```python
from build123d import *

# Parameters (mm, degrees)
SKETCH_1_R               = 2
EXTRUDE_1_DEPTH          = 4
SKETCH_1_3_W             = 3
SKETCH_1_3_H             = 52.773364798
EXTRUDE_2_DEPTH          = 34
CUT_EXTRUDE_1_DEPTH      = 174.554268557
CUT_EXTRUDE_1_DEPTH_BACK = 174.554268557
SKETCH_2_R               = 2.5


with BuildPart() as part:
    # Sketch 1 → Extrude 1 (new body)
    with BuildSketch(Plane(origin=(0, 0, 0), x_dir=(1, 0, 0), z_dir=(0, 1, 0))):
        Polygon((0, 0), (140, 0), (140, 44), (97, 44), (97, 96.773364798), (43, 96.773364798), (43, 44), (0, 44), align=None)
        with Locations(Location((8.8, 7, 0), (0, 0, 270))):
            Circle(SKETCH_1_R, mode=Mode.SUBTRACT)
        with Locations(Location((33.8, 7, 0), (0, 0, 270))):
            Circle(SKETCH_1_R, mode=Mode.SUBTRACT)
        with Locations(Location((8.8, 37, 0), (0, 0, 270))):
            Circle(SKETCH_1_R, mode=Mode.SUBTRACT)
        with Locations(Location((33.8, 37, 0), (0, 0, 270))):
            Circle(SKETCH_1_R, mode=Mode.SUBTRACT)
        with Locations(Location((131.2, 37, 0), (0, 0, 270))):
            Circle(SKETCH_1_R, mode=Mode.SUBTRACT)
        with Locations(Location((106.2, 7, 0), (0, 0, 270))):
            Circle(SKETCH_1_R, mode=Mode.SUBTRACT)
        with Locations(Location((131.2, 7, 0), (0, 0, 270))):
            Circle(SKETCH_1_R, mode=Mode.SUBTRACT)
        with Locations(Location((106.2, 37, 0), (0, 0, 270))):
            Circle(SKETCH_1_R, mode=Mode.SUBTRACT)
    extrude(amount=EXTRUDE_1_DEPTH)

    # Sketch 1_3 → Extrude 2 (add)
    with BuildSketch(Plane(origin=(0, 0, 0), x_dir=(1, 0, 0), z_dir=(0, 1, 0))):
        with Locations((98.5, 70.386682399)):
            Rectangle(SKETCH_1_3_W, SKETCH_1_3_H)
        with Locations((41.5, 70.386682399)):
            Rectangle(SKETCH_1_3_W, SKETCH_1_3_H)
    extrude(amount=EXTRUDE_2_DEPTH)

    # Sketch 2 → Cut-Extrude 1 (cut, two sides: drawn at the far end of the back side and taken through both)
    with BuildSketch(Plane(origin=(0, 0, 0), x_dir=(0, 0, -1), z_dir=(1, 0, 0)).offset(-CUT_EXTRUDE_1_DEPTH_BACK)):
        with Locations((51.5, 7.5)):
            Circle(SKETCH_2_R)
        with Locations((89.273364798, 7.5)):
            Circle(SKETCH_2_R)
        with Locations((89.273364798, 26.5)):
            Circle(SKETCH_2_R)
        with Locations((51.5, 26.5)):
            Circle(SKETCH_2_R)
    extrude(amount=CUT_EXTRUDE_1_DEPTH + CUT_EXTRUDE_1_DEPTH_BACK, mode=Mode.SUBTRACT)


solid = part.part
```
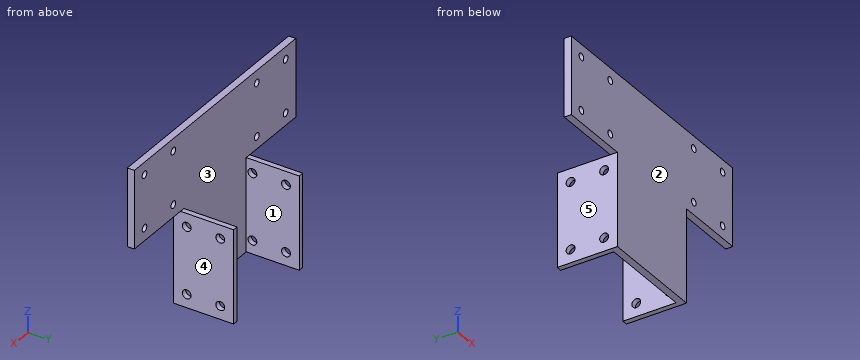
Work out the finished part from the listing and answer in its coordinate system (mm). Face numbers are marked on the shaded views. A direction names the side the tool comes from. Coordinates: 2 decimals unless noted, no trailing zeros. Loops run counter-clockwise (first coordinate to the right, second up) from the corner with the lowest first, then second, coordinate; pieces in that order, holes last.
1) Consider probe 1 along Z at (x, y) = (99.3, 26.5); probe 2 along Y at (x, z) = (99.25, -51.5); probe 3 along X at (y, z) = (2.85, -37). Determine where each line is inside the solid, lowest interval first.
Results:
probe 1: z = -96.77 to -91.77, -86.77 to -54, -49 to -44
probe 2: y = 0 to 5, 10 to 24, 29 to 34
probe 3: x = 0 to 6.8, 10.8 to 31.8, 35.8 to 104.2, 108.2 to 129.2, 133.2 to 140
2) Section B-B (y = 18.5) is taken. Give the vertices of the cut face in (x, z), plus the area to 3 significant figures.
Results:
outline: (40, -96.77) - (43, -96.77) - (43, -44) - (40, -44) - close; (97, -96.77) - (100, -96.77) - (100, -44) - (97, -44) - close
area: 317 mm2
3) For a pull along X with two mould halves and no side action, classify the marked faces 3, 4 and 5 as +X half, -X half, draft (parallel to the pull), parting line (faces both ways), or undercut.
Results:
face 3: undercut
face 4: +X half
face 5: -X half
4) Section D-D (y = 26.5) is taken. Give the vertices of the cut face in (x, z).
Results:
outline: (40, -96.77) - (43, -96.77) - (43, -91.77) - (40, -91.77) - close; (40, -86.77) - (43, -86.77) - (43, -54) - (40, -54) - close; (40, -49) - (43, -49) - (43, -44) - (40, -44) - close; (97, -96.77) - (100, -96.77) - (100, -91.77) - (97, -91.77) - close; (97, -86.77) - (100, -86.77) - (100, -54) - (97, -54) - close; (97, -49) - (100, -49) - (100, -44) - (97, -44) - close
5) Section A-A (z = -51.5) is taken. Give the vertices of the cut face in (x, y).
Results:
outline: (40, 0) - (100, 0) - (100, 5) - (97, 5) - (97, 4) - (43, 4) - (43, 5) - (40, 5) - close; (40, 10) - (43, 10) - (43, 24) - (40, 24) - close; (40, 29) - (43, 29) - (43, 34) - (40, 34) - close; (97, 10) - (100, 10) - (100, 24) - (97, 24) - close; (97, 29) - (100, 29) - (100, 34) - (97, 34) - close
6) Flat-ended cylindrical pins translate along their axes: pin 1 (10 mm diameter, centred on y = 25, z = -86, fed in from +X); pin 2 (3 mm diameter, centred on x = 54.5, z = -86, fed in from +Y); pin 3 (1.5 mm diameter, centred on x = 98, y = 13.5, fed in from +Z). Find the tip coordinate at first contact, or state that the pin passes through.
Results:
pin 1: stops at x = 100
pin 2: stops at y = 4
pin 3: stops at z = -44
7) For the marked faces 1 and 2, determine the directions among +Z, -Z, +X, -X, +Y, -Y from which every point of the face is accessible in a straight line to the end or side of a thin tool.
Results:
face 1: +Z, -Z, +Y
face 2: +Z, -Z, +X, -X, -Y
8) Section C-C (x = 131.2) is taken. Give the vertices of the cut face in (y, z).
Results:
outline: (0, -44) - (4, -44) - (4, -39) - (0, -39) - close; (0, -35) - (4, -35) - (4, -9) - (0, -9) - close; (0, -5) - (4, -5) - (4, 0) - (0, 0) - close
